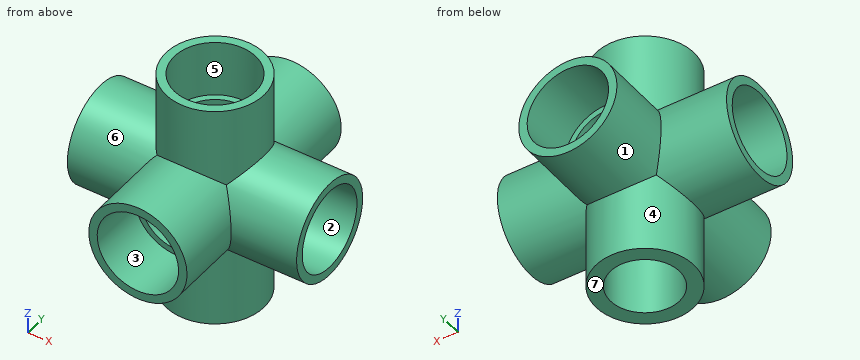
from build123d import *
from OCP.BRepAlgoAPI import BRepAlgoAPI_Cut
from OCP.TopTools import TopTools_ListOfShape
from build123d.topology import SkipClean

# Parameters (mm, degrees)
SKETCH_1_R                = 19.3
SKETCH_1_R_2              = 13.6
EXTRUDE_1_DEPTH           = 45.05
SKETCH_3_R                = 19.3
SKETCH_3_R_2              = 13.6
EXTRUDE_3_DEPTH           = 45.05
SKETCH_2_R                = 19.3
SKETCH_2_R_2              = 13.6
EXTRUDE_2_DEPTH           = 45.05
CUT_EXTRUDE_1_DEPTH       = 79.028889054
CUT_EXTRUDE_1_DEPTH_BACK  = 79.028889054
SKETCH_1_13_R             = 13.6
CUT_EXTRUDE_START         = -45.0500001
CUT_EXTRUDE_2_OUTLINE_R   = 13.6
CUT_EXTRUDE_2_DEPTH       = 90.1000002
CUT_EXTRUDE_3_DEPTH       = 79.028889054
CUT_EXTRUDE_3_DEPTH_BACK  = 124.078889054
CUT_EXTRUDE_3_START       = 45.05
SKETCH_2_8_R              = 13.6
CUT_EXTRUDE_START_2       = -45.05
SKETCH_1_15_R             = 16
CUT_EXTRUDE_4_DEPTH       = 22.2
CUT_EXTRUDE_START_3       = 45.05
SKETCH_1_16_R             = 16
CUT_EXTRUDE_5_DEPTH       = 22.2
SKETCH_3_9_R              = 16
CUT_EXTRUDE_6_DEPTH       = 22.2
SKETCH_3_10_R             = 16
CUT_EXTRUDE_7_DEPTH       = 22.2
CUT_EXTRUDE_START_4       = 22.85
CUT_EXTRUDE_8_OUTLINE_R   = 16
CUT_EXTRUDE_8_OUTLINE_R_2 = 13.6
CUT_EXTRUDE_8_DEPTH       = 22.2


with BuildPart() as part:
    # 草图1 → 凸台-拉伸1 (new, symmetric)
    with BuildSketch(Plane(origin=(0, 0, 0), x_dir=(1, 0, 0), z_dir=(0, 1, 0))):
        with Locations(Location((0, 0, 0), (0, 0, 270))):
            Circle(SKETCH_1_R)
        with Locations(Location((0, 0, 0), (0, 0, 270))):
            Circle(SKETCH_1_R_2, mode=Mode.SUBTRACT)
    extrude(amount=EXTRUDE_1_DEPTH, both=True)

    # 草图3 → 凸台-拉伸3 (add, symmetric)
    with BuildSketch(Plane(origin=(0, 0, 0), x_dir=(0, 0, -1), z_dir=(1, 0, 0))):
        with Locations(Location((0, 0, 0), (0, 0, 135))):
            Circle(SKETCH_3_R)
        with Locations(Location((0, 0, 0), (0, 0, 135.000001563))):
            Circle(SKETCH_3_R_2, mode=Mode.SUBTRACT)
    extrude(amount=EXTRUDE_3_DEPTH, both=True)

    # 草图2 → 凸台-拉伸2 (add, symmetric)
    with BuildSketch(Plane.XY):
        with Locations(Location((0, 0, 0), (0, 0, 225))):
            Circle(SKETCH_2_R)
        with Locations(Location((0, 0, 0), (0, 0, 224.999996387))):
            Circle(SKETCH_2_R_2, mode=Mode.SUBTRACT)
    extrude(amount=EXTRUDE_2_DEPTH, both=True)

    # 草图1<13> → 切除-拉伸1 (cut, two sides: drawn at the far end of the back side and taken through both)
    with BuildSketch(Plane(origin=(0, 0, 0), x_dir=(1, 0, 0), z_dir=(0, 1, 0)).offset(-CUT_EXTRUDE_1_DEPTH_BACK)):
        with Locations(Location((0, 0, 0), (0, 0, 270))):
            Circle(SKETCH_1_13_R)
    extrude(amount=CUT_EXTRUDE_1_DEPTH + CUT_EXTRUDE_1_DEPTH_BACK, mode=Mode.SUBTRACT)

    # 切除-拉伸2: read off the stored shape, not the designer's step
    # 切除-拉伸2 outline → 切除-拉伸2 (cut)
    with BuildSketch(Plane(origin=(0, 0, 0), x_dir=(0, 0, -1), z_dir=(1, 0, 0)).offset(CUT_EXTRUDE_START)):
        Circle(CUT_EXTRUDE_2_OUTLINE_R)
    extrude(amount=CUT_EXTRUDE_2_DEPTH, mode=Mode.SUBTRACT)

    # 草图2<8> → 切除-拉伸3 (cut, two sides: drawn at the far end of the back side and taken through both)
    with BuildSketch(Plane.XY.offset(CUT_EXTRUDE_3_START - CUT_EXTRUDE_3_DEPTH_BACK)):
        with Locations(Location((0, 0, 0), (0, 0, 225))):
            Circle(SKETCH_2_8_R)
    extrude(amount=CUT_EXTRUDE_3_DEPTH + CUT_EXTRUDE_3_DEPTH_BACK, mode=Mode.SUBTRACT)


with BuildPart() as cut_extrude_3_kept_piece:
    # of the separate pieces the step leaves, the one the design keeps (cut_extrude_3_pieces_kept)
    add(part.part.solids().sort_by_distance((0, -45.05, 19.3))[0])

    # 草图1<15> → 切除-拉伸4 (cut)
    with SkipClean():  # the faces are left unmerged after this step: merging them gives an invalid solid
        with BuildSketch(Plane(origin=(0, 0, 0), x_dir=(1, 0, 0), z_dir=(0, 1, 0)).offset(CUT_EXTRUDE_START_2)):
            with Locations(Location((0, 0, 0), (0, 0, 270))):
                Circle(SKETCH_1_15_R)
        extrude(amount=CUT_EXTRUDE_4_DEPTH, mode=Mode.SUBTRACT)

    # 草图1<16> → 切除-拉伸5 (cut)
    with SkipClean():  # the faces are left unmerged after this step: merging them gives an invalid solid
        with BuildSketch(Plane(origin=(0, 0, 0), x_dir=(1, 0, 0), z_dir=(0, 1, 0)).offset(CUT_EXTRUDE_START_3)):
            with Locations(Location((0, 0, 0), (0, 0, 270))):
                Circle(SKETCH_1_16_R)
        extrude(amount=-CUT_EXTRUDE_5_DEPTH, mode=Mode.SUBTRACT)

    # 草图3<9> → 切除-拉伸6 (cut)
    with SkipClean():  # the faces are left unmerged after this step: merging them gives an invalid solid
        with BuildSketch(Plane(origin=(0, 0, 0), x_dir=(0, 0, -1), z_dir=(1, 0, 0)).offset(CUT_EXTRUDE_START_2)):
            Circle(SKETCH_3_9_R)
        extrude(amount=CUT_EXTRUDE_6_DEPTH, mode=Mode.SUBTRACT)

    # 草图3<10> → 切除-拉伸7 (cut)
    with SkipClean():  # the faces are left unmerged after this step: merging them gives an invalid solid
        with BuildSketch(Plane(origin=(0, 0, 0), x_dir=(0, 0, -1), z_dir=(1, 0, 0)).offset(CUT_EXTRUDE_START_3)):
            Circle(SKETCH_3_10_R)
        extrude(amount=-CUT_EXTRUDE_7_DEPTH, mode=Mode.SUBTRACT)


with BuildPart() as cut_extrude_8_tool:
    # 切除-拉伸8: read off the stored shape, not the designer's step
    # 切除-拉伸8 outline → 切除-拉伸8 (new body)
    with BuildSketch(Plane.XY.offset(CUT_EXTRUDE_START_4)):
        Circle(CUT_EXTRUDE_8_OUTLINE_R)
        Circle(CUT_EXTRUDE_8_OUTLINE_R_2, mode=Mode.SUBTRACT)
    extrude(amount=CUT_EXTRUDE_8_DEPTH)


with BuildPart() as cut_extrude_3_kept_piece_1:
    add(cut_extrude_3_kept_piece.part)

    # 切除-拉伸8: cut by cut_extrude_8_tool, with a tolerance
    cut_extrude_8_stock = TopTools_ListOfShape()
    cut_extrude_8_stock.Append(cut_extrude_3_kept_piece_1.part.wrapped)
    cut_extrude_8_tools = TopTools_ListOfShape()
    cut_extrude_8_tools.Append(cut_extrude_8_tool.part.wrapped)
    cut_extrude_8_cut = BRepAlgoAPI_Cut()
    cut_extrude_8_cut.SetArguments(cut_extrude_8_stock)
    cut_extrude_8_cut.SetTools(cut_extrude_8_tools)
    cut_extrude_8_cut.SetFuzzyValue(0.00001)
    cut_extrude_8_cut.Build()
    add(Compound.cast(cut_extrude_8_cut.Shape()).solids(), mode=Mode.REPLACE)


solid = cut_extrude_3_kept_piece_1.part
Model file for the job. Use its own axes, mm. Face numbers are marked on the shaded views. A direction names the side the tool comes from. Give positions to 0.01 mm unless a question says otherwise; leave off trailing zeros. Loops run counter-clockwise (first coordinate to the right, second up) from the corner with the lowest first, then second, coordinate; pieces in that order, holes last. Notation, with made-up numbers: (76, -27.5) - (107, -27.5) arc R14 ccw to (107, -10.5) - close; hole circle Ø5 at (53.25, 14). An arc over 180 degrees is marked (long way). Use one line per item in the form item = value.
(1) 3-axis set-ups, long thin cutter, end or side, ignore diameter. For the marked faces 1, 2, 3 and 4: which of +Z, -Z, +X, -X, +Y, -Y reach the whole face in a straight line?
Determined:
face_1 = +Y
face_2 = +X
face_3 = -Y
face_4 = -Z
(2) Drill centre lines: L1, parallel to X at y = 0, z = 21.75; L2, parallel to X at y = -14.5, z = 0; L3, parallel to Z at x = -18.5, y = 0. Where is each one in solid material? Low to high.
Determined:
L1 = -19.3 to -13.6, 13.6 to 19.3
L2 = -22.85 to -13.6, 13.6 to 22.85
L3 = -45.05 to -13.6, 13.6 to 45.05
(3) Cut at A-A (x = 21.5). Give the cut face in (y, z), then the cut area to 3 significant figures.
Determined:
outline = circle Ø38.6 at (0, 0); hole circle Ø27.2 at (0, 0)
area = 589 mm^2
(4) Pull direction Y, two halves, no side cores. Call the marked faces 5, 6 and 7: pulls with the +Y half, pulls with the -Y half, needs draft (parallel to the pull), parting line crosses it, or undercut.
Determined:
face_5 = undercut
face_6 = parting line crosses it
face_7 = needs draft
(5) Cut at C-C (z = 0). Count the separate pieces of the cut face and the enclosed holes in it, then the cut area to 3 significant figures.
Determined:
separate_pieces = 4
enclosed_holes = 0
area = 878 mm^2
(6) Drop flat-ended pins along their axis: P1, Ø2, axis at x = -6, z = 32.5, coming from the -Y side; P2, Ø10, axis at y = -25.5, z = -8.5, coming from the +X side; P3, Ø4, axis at x = 29.5, y = -17, coming from the +Z side. Give the stop position or say it passes through.
Determined:
P1 = -18.64
P2 = 18.98
P3 = 12.14
